Could you check a few things on this drawing? It's one solid part, dimensions in mm from its lowest x, y, z. Give positions to 0.01 mm unless a question says otherwise; leave off trailing zeros. Order: outer loops, then holes, each group sorted by start corner. A loop starts at its lowest first (then second) coordinate and runs counter-clockwise, first axis right, second up. Notation, with made-up numbers: (60, 26.5) - (106, 26.5) arc R15 ccw to (106, 38.5) - close; hole circle Ø1 at (55, -7). An arc over 180 degrees is marked (long way). Return JSON: item names as keys, results as strings.
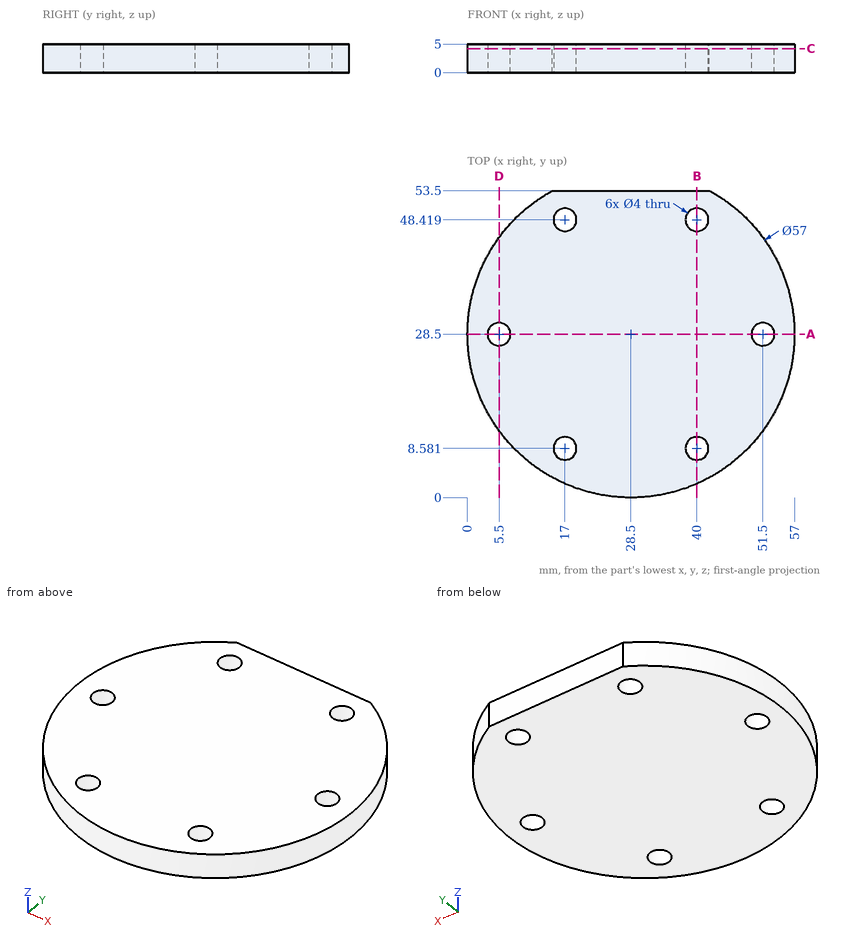
1. For pin 1 Ø2.5 at (x, y) = (40, 8.58) entering from -Z; pin 2 Ø1 at (y, z) = (25.5, 0.5) entering from -X; pin 3 Ø1.5 at (x, z) = (46, 3.5) entering from -Y; pin 4 Ø1.5 at (y, z) = (45.5, 3.5) entering from -X, each with a flat end and sliding along its axis, tell me the tip position at first contact or that it passes through.
Checks:
{"pin 1": "through", "pin 2": "x = 0.11", "pin 3": "y = 5.44", "pin 4": "x = 5.09"}
2. Suppose I cut it at C-C (z = 4.2). List the corners of the cut face in (x, y) for me.
Checks:
{"outline": "(14.82, 53.5) arc R28.5 ccw (long way) to (42.18, 53.5) - close; hole circle Ø4 at (5.5, 28.5); hole circle Ø4 at (17, 8.58); hole circle Ø4 at (17, 48.42); hole circle Ø4 at (40, 8.58); hole circle Ø4 at (40, 48.42); hole circle Ø4 at (51.5, 28.5)"}
3. Suppose I cut it at B-B (x = 40). List the corners of the cut face in (y, z) for me.
Checks:
{"outline": "(2.42, 0) - (6.58, 0) - (6.58, 5) - (2.42, 5) - close; (10.58, 0) - (46.42, 0) - (46.42, 5) - (10.58, 5) - close; (50.42, 0) - (53.5, 0) - (53.5, 5) - (50.42, 5) - close"}
4. If I drill on L1, parallel to X at y = 7, z = 2.9 (1 decimal); L2, parallel to X at y = 9.5, z = 1.4 (1 decimal); L3, parallel to Y at x = 40, z = 1.3, over which ranges is the centre line in solid material (lowest first)? Write a range as [from, to].
Checks:
{"L1": "[9.8, 15.8], [18.2, 38.8], [41.2, 47.2]", "L2": "[7.3, 15.2], [18.8, 38.2], [41.8, 49.7]", "L3": "[2.42, 6.58], [10.58, 46.42], [50.42, 53.5]"}
5. Suppose I cut it at D-D (x = 5.5). List the corners of the cut face in (y, z) for me.
Checks:
{"outline": "(11.67, 0) - (26.5, 0) - (26.5, 5) - (11.67, 5) - close; (30.5, 0) - (45.33, 0) - (45.33, 5) - (30.5, 5) - close"}
6. Suppose I cut it at A-A (y = 28.5). List the corners of the cut face in (x, z) for me, plus the area to 3 significant figures.
Checks:
{"outline": "(0, 0) - (3.5, 0) - (3.5, 5) - (0, 5) - close; (7.5, 0) - (49.5, 0) - (49.5, 5) - (7.5, 5) - close; (53.5, 0) - (57, 0) - (57, 5) - (53.5, 5) - close", "area": "245 mm^2"}
